Part model, mm, in its own coordinate system. Give positions to 0.01 mm unless a question says otherwise; leave off trailing zeros. Write each loop counter-clockwise with the first axis right and the second up, starting at its lowest first coordinate (ties: lowest second). Pieces come first, ordered by that corner, then holes.
Autodesk Inventor part; units mm, degrees
ref_plane "YZ Plane" through (0, 0, 0) normal (1, 0, 0) x (0, 1, 0)
ref_plane "XZ Plane" through (0, 0, 0) normal (0, 1, 0) x (-1, 0, 0)
ref_plane "XY Plane" through (0, 0, 0) normal (0, 0, 1) x (1, 0, 0)
sketch "Sketch2" plane through (0, 0, 0) normal (0, 0, 1) x (1, 0, 0)
  circle A0 centre (5, 90) radius 3
  circle A1 centre (133, 5) radius 3
  circle A2 centre (133, 90) radius 3
  line L0 (0, 0) -> (138, 0)
  line L1 (138, 0) -> (138, 96)
  line L2 (138, 96) -> (0, 96)
  line L3 (0, 96) -> (0, 0)
  circle A3 centre (6, 20) radius 2
  circle A4 centre (6, 66) radius 2
  circle A5 centre (122, 40) radius 2
extrude "Extrusion2" add sketch "Sketch2" along normal mid plane 2 contours L3 L2 L1 L0 | A3 | A4 | A5
sketch "Sketch3" plane through (0, 0, 1) normal (0, 0, 1) x (1, 0, 0)
  circle A0 centre (6, 20) radius 2 construction
  circle A1 centre (6, 20) radius 0.5
  point P0 (0, 0)
  dimension "d4" = 1
extrude "Extrusion3" [suppressed]
sketch "Sketch4" plane through (0, 0, 1) normal (0, 0, 1) x (1, 0, 0)
  circle A0 centre (6, 66) radius 2
  circle A1 centre (6, 66) radius 0.5
  point P0 (0, 0)
  dimension "d7" = 1
extrude "Extrusion4" [suppressed]
sketch "Sketch5" plane through (0, 0, 1) normal (0, 0, 1) x (1, 0, 0)
  circle A0 centre (122, 40) radius 2
  circle A1 centre (122, 40) radius 0.5
  point P0 (0, 0)
  dimension "d10" = 1
extrude "Extrusion5" [suppressed]
ref_plane "Work Plane1" through (64, 0, 1) normal (-1, 0, 0) x (0, 0, 1)
ref_plane "Work Plane2" through (0, 43, 1) normal (0, -1, 0) x (1, 0, 0)
sketch "Sketch7" plane through (0, 0, 1) normal (0, 0, 1) x (1, 0, 0)
  line L0 (39, 7) -> (89, 7)
  line L1 (89, 7) -> (89, 5)
  line L2 (89, 5) -> (39, 5)
  line L3 (39, 5) -> (39, 7)
  line L4 (64, -19.2) -> (64, 115.2) construction
  line L5 (165.6, 43) -> (-27.6, 43) construction
  line L6 (0, 0) -> (138, 0)
  line L7 (8, 68) -> (10, 68)
  line L8 (10, 68) -> (10, 18)
  line L9 (10, 18) -> (8, 18)
  line L10 (8, 18) -> (8, 68)
  line L11 (0, 96) -> (0, 0)
  line L12 (118, 68) -> (120, 68)
  line L13 (120, 68) -> (120, 18)
  line L14 (120, 18) -> (118, 18)
  line L15 (118, 18) -> (118, 68)
  line L16 (39, 80) -> (89, 80)
  line L17 (89, 80) -> (89, 78)
  line L18 (89, 78) -> (39, 78)
  line L19 (39, 78) -> (39, 80)
  point P0 (64, 7)
  point P1 (10, 43)
  point P2 (118, 43)
  point P3 (64, 78)
  dimension "d15" = 2
  dimension "d16" = 5
  dimension "d17" = 50
  dimension "d18" = 2
  dimension "d19" = 50
  dimension "d20" = 8
  dimension "d23" = 50
  dimension "d24" = 2
  dimension "d25" = 118
  dimension "d26" = 2
  dimension "d27" = 50
  dimension "d28" = 78
extrude "Extrusion6" cut sketch "Sketch7" against normal through all
properties part number "mount_plate"
1) Saw through at B-B (x = 5). Write the cut outline in (y, z), and give its area (3 significant figures).
Check result:
outline: (0, -1) - (87, -1) - (87, 1) - (0, 1) - close; (93, -1) - (96, -1) - (96, 1) - (93, 1) - close
area: 180 mm2
2) Saw through at C-C (x = 70). Write the cut outline in (y, z).
Check result:
outline: (0, -1) - (5, -1) - (5, 1) - (0, 1) - close; (7, -1) - (78, -1) - (78, 1) - (7, 1) - close; (80, -1) - (96, -1) - (96, 1) - (80, 1) - close
3) Saw through at D-D (z = 0.6). Write the cut outline in (x, y), and give its area (3 significant figures).
Check result:
outline: (0, 0) - (138, 0) - (138, 96) - (0, 96) - close; hole circle Ø6 at (5, 90); hole (8, 18) - (10, 18) - (10, 68) - (8, 68) - close; hole (39, 5) - (89, 5) - (89, 7) - (39, 7) - close; hole (39, 78) - (89, 78) - (89, 80) - (39, 80) - close; hole (118, 18) - (120, 18) - (120, 68) - (118, 68) - close; hole circle Ø6 at (133, 5); hole circle Ø6 at (133, 90)
area: 12,800 mm2
4) Drill centre lines: L1, parallel to X at y = 30.5, z = 0.45; L2, parallel to Y at x = 74.5, z = -0.8; L3, parallel to Y at x = 133, z = 0.05. Where is each one in solid material? Low to high.
Check result:
L1: x = 0 to 8, 10 to 118, 120 to 138
L2: y = 0 to 5, 7 to 78, 80 to 96
L3: y = 0 to 2, 8 to 87, 93 to 96
5) Mould opens along Y. For faces 1 (the cylindrical face through (135.86, 5.9, 0.01)), 2 (the flat face through (68, 49, -1)) say: +Y half, -Y half, draft (parallel to the pull), parting line (faces both ways), or undercut.
Check result:
face 1: undercut
face 2: draft
6) Saw through at A-A (y = 19.5). Write the cut outline in (x, z), and give its area (3 significant figures).
Check result:
outline: (0, -1) - (8, -1) - (8, 1) - (0, 1) - close; (10, -1) - (118, -1) - (118, 1) - (10, 1) - close; (120, -1) - (138, -1) - (138, 1) - (120, 1) - close
area: 268 mm2
